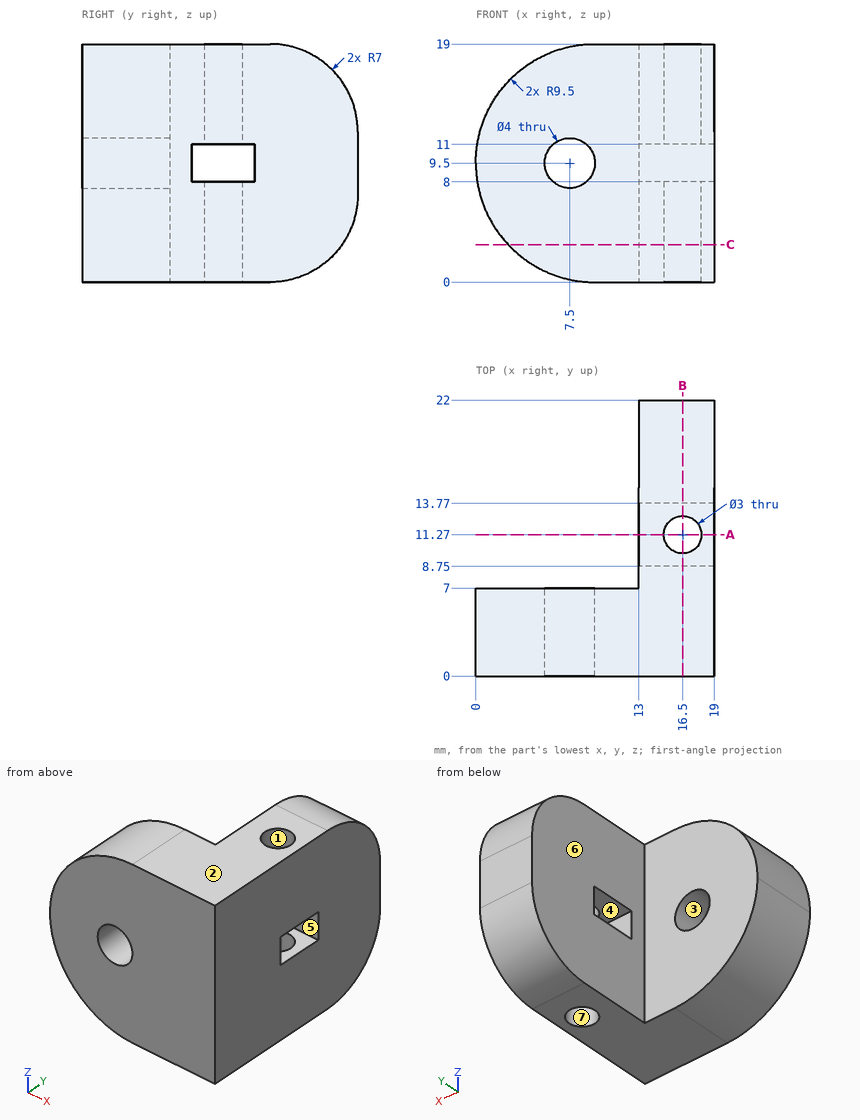
Part print with two shaded views. Sizes in mm from the minimum x, y, z corner. A direction names the side the tool comes from. Round coordinates to 2 decimals unless told otherwise and drop trailing zeros. Order: outer loops, then holes, each group sorted by start corner. A loop starts at its lowest first (then second) coordinate and runs counter-clockwise, first axis right, second up. Notation, with made-up numbers: M 12.5,11 L 39.5,11 A32 ccw 39.5,46 Z; hole C -30,35 d2. An arc over 180 degrees is marked long. Answer in a Markdown table with one row per item. Add a question column.
Q1. Cut at C-C on z = 3. Give the cut face in (x, y).
Q2. Mould opens along Z. For the marked faces 1, 2, 3 and 4 say: +Z half, -Z half, draft (parallel to the pull), parting line (faces both ways), or undercut.
Q3. Wall check: L1, parallel to X at y = 2.25, z = 9.5; L2, parallel to Z at x = 14.75, y = 11; L3, parallel to X at y = 11.27, z = 15.75. Give the ranges that are in metal, low to high. Write a range as from..to.
Q4. 3-axis set-ups, long thin cutter, end or side, ignore diameter. For the marked faces 5, 6 and 7: which of +Z, -Z, +X, -X, +Y, -Y reach the whole face in a straight line?
Q5. Pin check, flat tips, straight feed: pin 1 (2 mm diameter, centred on x = 15, z = 16, fed in from +Y); pin 2 (4 mm diameter, centred on x = 16.5, y = 11.27, fed in from -Z); pin 3 (7.5 mm diameter, centred on y = 12.5, z = 6, fed in from -X); pin 4 (2 mm diameter, centred on x = 13, z = 5.5, fed in from +Y). Stop position of each tip, or through.
Q6. Cut at B-B on x = 16.5. Give the cut face in (y, z), and give its area (3 significant figures).
Q7. Cut at A-A on y = 11.27. Give the cut face in (x, z).
Established:
| question | item | result |
|---|---|---|
| 1 | outline | M 2.57,0 L 19,0 L 19,20.74 L 13,20.74 L 13,7 L 2.57,7 Z; hole C 16.5,11.27 d3 |
| 2 | face 1 | draft |
| 2 | face 2 | +Z half |
| 2 | face 3 | undercut |
| 2 | face 4 | undercut |
| 3 | L1 | x = 0..5.5, 9.5..19 |
| 3 | L2 | z = 0..8, 11..19 |
| 3 | L3 | x = 13..15, 18..19 |
| 4 | face 5 | +X, -X |
| 4 | face 6 | +Z, -Z, -X, +Y |
| 4 | face 7 | +Z, -Z |
| 5 | pin 1 | stops at y = 21.32 |
| 5 | pin 2 | stops at z = 0 |
| 5 | pin 3 | stops at x = 13 |
| 5 | pin 4 | stops at y = 21.98 |
| 6 | outline | M 0,0 L 9.77,0 L 9.77,8 L 8.75,8 L 8.75,11 L 9.77,11 L 9.77,19 L 0,19 Z; M 12.77,0 L 15,0 A7 ccw 22,7 L 22,12 A7 ccw 15,19 L 12.77,19 L 12.77,11 L 13.77,11 L 13.77,8 L 12.77,8 Z |
| 6 | area | 334 mm2 |
| 7 | outline | M 13,0 L 15,0 L 15,8 L 13,8 Z; M 13,11 L 15,11 L 15,19 L 13,19 Z; M 18,0 L 19,0 L 19,8 L 18,8 Z; M 18,11 L 19,11 L 19,19 L 18,19 Z |
